from build123d import *

# Parameters (mm, degrees)
SKETCH1_W                          = 80
SKETCH1_H                          = 85
SKETCH1_R                          = 20
SKETCH1_R_2                        = 2.75
FRONT_PLATE_DEPTH                  = 8
BENCH_FOOT_START                   = -20
SKETCH2_W                          = 80
SKETCH2_H                          = 8
BENCH_FOOT_DEPTH                   = 70
FOUR_M6_FOOT_CLEARANCES_DEPTH      = 82.240384046
FOUR_M6_FOOT_CLEARANCES_DEPTH_BACK = 82.240384046
SKETCH3_R                          = 3.3


with BuildPart() as part:
    # Sketch1 → Front_Plate (new body)
    with BuildSketch(Plane.XY):
        with Locations((0, -7.5)):
            Rectangle(SKETCH1_W, SKETCH1_H)
        Circle(SKETCH1_R, mode=Mode.SUBTRACT)
        with Locations((-23.55, -23.55)):
            Circle(SKETCH1_R_2, mode=Mode.SUBTRACT)
        with Locations((-23.55, 23.55)):
            Circle(SKETCH1_R_2, mode=Mode.SUBTRACT)
        with Locations((23.55, -23.55)):
            Circle(SKETCH1_R_2, mode=Mode.SUBTRACT)
        with Locations((23.55, 23.55)):
            Circle(SKETCH1_R_2, mode=Mode.SUBTRACT)
    extrude(amount=FRONT_PLATE_DEPTH)

    # Sketch2 → Bench_Foot (add)
    with BuildSketch(Plane.XY.offset(BENCH_FOOT_START)):
        with Locations((0, -46)):
            Rectangle(SKETCH2_W, SKETCH2_H)
    extrude(amount=BENCH_FOOT_DEPTH)

    # Sketch3 → Four_M6_Foot_Clearances (cut, two sides: drawn at the far end of the back side and taken through both)
    with BuildSketch(Plane(origin=(0, 0, 0), x_dir=(1, 0, 0), z_dir=(0, 1, 0)).offset(-FOUR_M6_FOOT_CLEARANCES_DEPTH_BACK)):
        with Locations(Location((-28, 10, 0), (0, 0, 270))):
            Circle(SKETCH3_R)
        with Locations(Location((-28, -38, 0), (0, 0, 270))):
            Circle(SKETCH3_R)
        with Locations(Location((28, 10, 0), (0, 0, 270))):
            Circle(SKETCH3_R)
        with Locations(Location((28, -38, 0), (0, 0, 270))):
            Circle(SKETCH3_R)
    extrude(amount=FOUR_M6_FOOT_CLEARANCES_DEPTH + FOUR_M6_FOOT_CLEARANCES_DEPTH_BACK, mode=Mode.SUBTRACT)


solid = part.part
Work out the finished part from the listing and answer in its coordinate system (mm). A direction names the side the tool comes from. Give positions to 0.01 mm unless a question says otherwise; leave off trailing zeros. Loops run counter-clockwise (first coordinate to the right, second up) from the corner with the lowest first, then second, coordinate; pieces in that order, holes last. Notation, with made-up numbers: (78, -40) -> (82, -40) arc R23 ccw to (82, -7) -> close; hole circle Ø5 at (-1, -18.5). An arc over 180 degrees is marked (long way). Use a Markdown table: item, result. Add a question column.
1) Which of the six approach directions +Z, -Z, +X, -X, +Y, -Y give full straight-line access (tool end or side, diameter ignored) to faces 4 (the flat face through (-9, -20, 8)), 5 (the flat face through (-9, -20, 0)), 6 (the cylindrical face through (-4.336, -19.524, 3.944))?
2) The part is cut by section B-B, the plane x = 23.55. Determine the outline of the cut face in (y, z), plus the area to 3 significant figures.
3) The part is cut by section C-C, the plane y = 23.55. Determine the outline of the cut face in (x, z).
4) Each of these flat-tipped pins is pushed along its axis until it touches: P1, Ø9, axis at x = 23.55, y = 23.55, coming from the +Z side; P2, Ø16, axis at x = 15, z = -11.5, coming from the +Y side; P3, Ø1.5, axis at x = 31.5, y = 2.5, coming from the -Z side; P4, Ø4.5, axis at x = 23.55, y = -23.55, coming from the -Z side. Where does it stop, or does it pass through?
5) The part is cut by section D-D, the plane y = 0. Determine the outline of the cut face in (x, z).
6) The part is cut by section A-A, the plane z = -10. Determine the outline of the cut face in (x, y), plus the area to 3 significant figures.
7) Consider line 1 along Z through (x, y) = (28, -46.75); line 2 along X through (y, z) = (-44, 38); line 3 along Y through (x, z) = (-23.55, 6.25). Determine where each line is inside the solid, lowest interval first.
8) For a pull along Z with two mould halves and no side action, classify faces 1 (the cylindrical face through (-25.77, -46.06, 35.57)), 2 (the flat face through (-1, -42, 29)), 3 (the flat face through (-1, -46, -20)) as +Z half, -Z half, draft (parallel to the pull), parting line (faces both ways), or undercut.
Reported:
| question | item | result |
|---|---|---|
| 1 | face 4 | +Z, +X, -X, +Y |
| 1 | face 5 | -Z, +X, -X, +Y |
| 1 | face 6 | +Z, -Z |
| 2 | outline | (-50, -20) -> (-42, -20) -> (-42, 0) -> (-26.3, 0) -> (-26.3, 8) -> (-42, 8) -> (-42, 50) -> (-50, 50) -> close; (-20.8, 0) -> (20.8, 0) -> (20.8, 8) -> (-20.8, 8) -> close; (26.3, 0) -> (35, 0) -> (35, 8) -> (26.3, 8) -> close |
| 2 | area | 1,090 mm^2 |
| 3 | outline | (-40, 0) -> (-26.3, 0) -> (-26.3, 8) -> (-40, 8) -> close; (-20.8, 0) -> (20.8, 0) -> (20.8, 8) -> (-20.8, 8) -> close; (26.3, 0) -> (40, 0) -> (40, 8) -> (26.3, 8) -> close |
| 4 | P1 | stops at z = 8 |
| 4 | P2 | stops at y = -42 |
| 4 | P3 | stops at z = 0 |
| 4 | P4 | passes through |
| 5 | outline | (-40, 0) -> (-20, 0) -> (-20, 8) -> (-40, 8) -> close; (20, 0) -> (40, 0) -> (40, 8) -> (20, 8) -> close |
| 6 | outline | (-40, -50) -> (-31.3, -50) -> (-31.3, -42) -> (-40, -42) -> close; (-24.7, -50) -> (24.7, -50) -> (24.7, -42) -> (-24.7, -42) -> close; (31.3, -50) -> (40, -50) -> (40, -42) -> (31.3, -42) -> close |
| 6 | area | 534 mm^2 |
| 7 | line 1 | z = -20 to -13.3, -6.7 to 34.7, 41.3 to 50 |
| 7 | line 2 | x = -40 to -31.3, -24.7 to 24.7, 31.3 to 40 |
| 7 | line 3 | y = -50 to -26.3, -20.8 to 20.8, 26.3 to 35 |
| 8 | face 1 | undercut |
| 8 | face 2 | draft |
| 8 | face 3 | -Z half |
